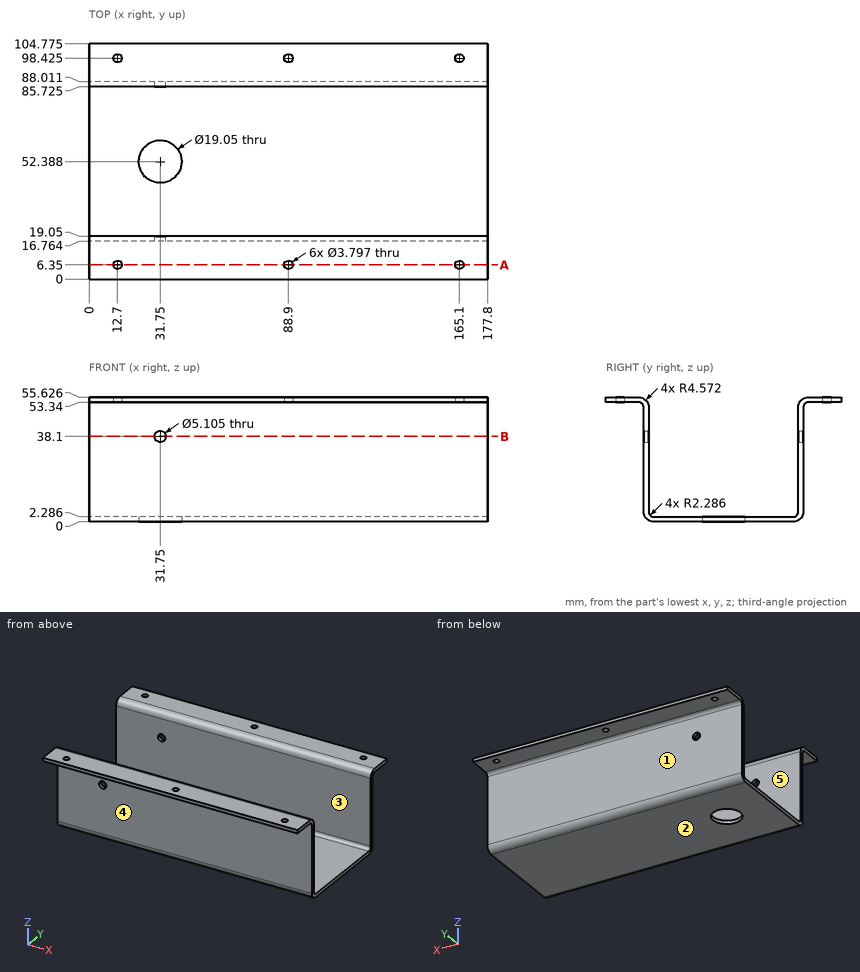
The drawing under review shows one solid part. Ordinate dimensions are in mm from its lowest x, y, z. A direction names the side the tool comes from. Round coordinates to 2 decimals unless told otherwise and drop trailing zeros. Write each loop counter-clockwise with the first axis right and the second up, starting at its lowest first coordinate (ties: lowest second). Pieces come first, ordered by that corner, then holes.
(1) Insertion check: pin 1 (11.5 mm diameter, centred on x = 61, y = 9, fed in from -Z); pin 2 (3 mm diameter, centred on x = 124, y = 16.5, fed in from -Z) (1 decimal); pin 3 (5 mm diameter, centred on x = 122, z = 11, fed in from +Y); pin 4 (3 mm diameter, centred on x = 88.9, y = 6.35, fed in from +Z). Each pin has a flat end and moves straight along its axis. Give the tip position at first contact, or say it passes through.
(2) We need section B-B on z = 38.1. Give the number of separate pieces and of enclosed holes in the cut face.
(3) Machinability: for the marked faces 4 and 5, which of the approach directions +Z, -Z, +X, -X, +Y, -Y give a long, thin tool a straight path to every point of the face, cutting with its end or side? Answer none if there is none.
(4) Mouldability with a two-part tool opening along Y and no side actions: class the marked faces 1, 2 and 3 as +Y half, -Y half, draft (parallel to the pull), parting line (faces both ways), or undercut.
(5) Wall thickness on L1, parallel to Y at x = 12, z = 54 (1 decimal); L2, parallel to Z at x = 115.5, y = 38 (1 decimal); L3, parallel to Z at x = 118.5, y = 10 (1 decimal): over which ranges is each line inside the solid? List them lowest first.
(6) We need section A-A on y = 6.35. Give the boundary of the cut face in (x, z) (1 decimal).
Findings below:
1. pin 1: stops at z = 53.32
1. pin 2: stops at z = 1.4
1. pin 3: stops at y = 88.01
1. pin 4: passes through
2. separate pieces: 4
2. enclosed holes: 0
3. face 4: -Z, +X, -X, -Y
3. face 5: +Z, +X, -X
4. face 1: +Y half
4. face 2: draft
4. face 3: undercut
5. L1: y = 0 to 4.6, 8.1 to 18, 86.8 to 96.7, 100.2 to 104.8
5. L2: z = 0 to 2.3
5. L3: z = 53.3 to 55.6
6. outline: (0, 53.3) - (10.8, 53.3) - (10.8, 55.6) - (0, 55.6) - close; (14.6, 53.3) - (87, 53.3) - (87, 55.6) - (14.6, 55.6) - close; (90.8, 53.3) - (163.2, 53.3) - (163.2, 55.6) - (90.8, 55.6) - close; (167, 53.3) - (177.8, 53.3) - (177.8, 55.6) - (167, 55.6) - close
